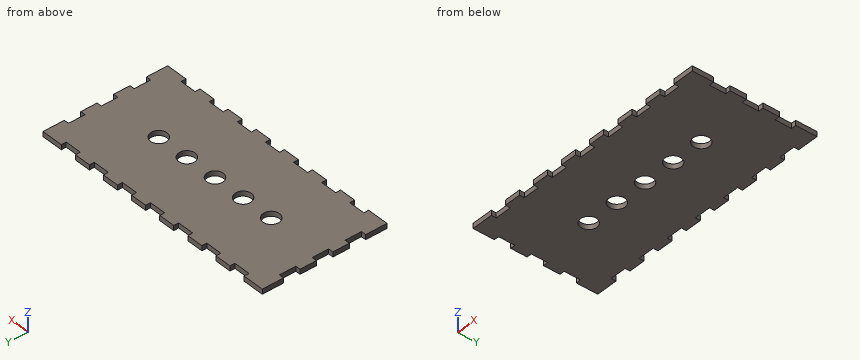
```python
from build123d import *

# Parameters (mm, degrees)
SKETCH1_R           = 5
BOSS_EXTRUDE1_DEPTH = 3


with BuildPart() as part:
    # Sketch1 → Boss-Extrude1 (new body)
    with BuildSketch(Plane.XY):
        Polygon((0, 60), (0, 50), (-3, 50), (-3, 40), (0, 40), (0, 30), (-3, 30), (-3, 20), (0, 20), (0, 10), (-3, 10), (-3, 0), (-3, -3), (0, -3), (10, -3), (10, 0), (20, 0), (20, -3), (30, -3), (30, 0), (40, 0), (40, -3), (50, -3), (50, 0), (60, 0), (60, -3), (70, -3), (70, 0), (80, 0), (80, -3), (90, -3), (90, 0), (100, 0), (100, -3), (110, -3), (110, 0), (120, 0), (120, -3), (130, -3), (130, 0), (140, 0), (140, -3), (150, -3), (153, -3), (153, 0), (153, 10), (150, 10), (150, 20), (153, 20), (153, 30), (150, 30), (150, 40), (153, 40), (153, 50), (150, 50), (150, 60), (153, 60), (153, 70), (153, 73), (150, 73), (140, 73), (140, 70), (130, 70), (130, 73), (120, 73), (120, 70), (110, 70), (110, 73), (100, 73), (100, 70), (90, 70), (90, 73), (80, 73), (80, 70), (70, 70), (70, 73), (60, 73), (60, 70), (50, 70), (50, 73), (40, 73), (40, 70), (30, 70), (30, 73), (20, 73), (20, 70), (10, 70), (10, 73), (0, 73), (-3, 73), (-3, 70), (-3, 60), align=None)
        with Locations((35, 35)):
            Circle(SKETCH1_R, mode=Mode.SUBTRACT)
        with Locations((55, 35)):
            Circle(SKETCH1_R, mode=Mode.SUBTRACT)
        with Locations((75, 35)):
            Circle(SKETCH1_R, mode=Mode.SUBTRACT)
        with Locations((95, 35)):
            Circle(SKETCH1_R, mode=Mode.SUBTRACT)
        with Locations((115, 35)):
            Circle(SKETCH1_R, mode=Mode.SUBTRACT)
    extrude(amount=BOSS_EXTRUDE1_DEPTH)


solid = part.part
```
Can you work these out from the model? Positions are in its coordinate system, mm. Give positions to 0.01 mm unless a question says otherwise; leave off trailing zeros. Loops run counter-clockwise (first coordinate to the right, second up) from the corner with the lowest first, then second, coordinate; pieces in that order, holes last. Notation, with made-up numbers: M 20,87.25 L 62,87.25 A19 cw 62,115.25 Z; hole C -28,-27 d1. An arc over 180 degrees is marked long. Use one line per item in the form item = value. Start each with the question number.
(1) I want a section at A-A, the plane x = 95. Write out the boundary of the cut face in (y, z), and give its area (3 significant figures).
(2) Please list where these lines run through material, in increasing order: line 1 (Y direction, x = 55, z = 1.2); line 2 (X direction, y = 32, z = 1.8); line 3 (X direction, y = 52.5, z = 2.6).
(3) I'm going to push flat-ended pins straight in: P1, Ø0.9, axis at x = 53, z = 1, coming from the +Y side; P2, Ø0.9, axis at x = 93.5, z = 1, coming from the -Y side. Where does each tip first touch, or does it pass through?
(4) I want a section at B-B, the plane y = 35. Write out the boundary of the cut face in (x, z), and give its area (3 significant figures).
(5) I want a section at C-C, the plane z = 1.25. State how many separate pieces and enclosed holes the cut face has, and give its area (3 significant figures).
(6) I want a section at D-D, the plane x = 38.5. Write out the boundary of the cut face in (y, z), and give its area (3 significant figures).
Worked out:
q1.outline = M 0,0 L 30,0 L 30,3 L 0,3 Z; M 40,0 L 70,0 L 70,3 L 40,3 Z
q1.area = 180 mm²
q2.line_1 = 0 to 30, 40 to 70
q2.line_2 = 0 to 31, 39 to 51, 59 to 71, 79 to 91, 99 to 111, 119 to 150
q2.line_3 = 0 to 150
q3.P1 = 70
q3.P2 = 0
q4.outline = M 0,0 L 30,0 L 30,3 L 0,3 Z; M 40,0 L 50,0 L 50,3 L 40,3 Z; M 60,0 L 70,0 L 70,3 L 60,3 Z; M 80,0 L 90,0 L 90,3 L 80,3 Z; M 100,0 L 110,0 L 110,3 L 100,3 Z; M 120,0 L 150,0 L 150,3 L 120,3 Z
q4.area = 300 mm²
q5.separate_pieces = 1
q5.enclosed_holes = 5
q5.area = 10,900 mm²
q6.outline = M 0,0 L 31.43,0 L 31.43,3 L 0,3 Z; M 38.57,0 L 70,0 L 70,3 L 38.57,3 Z
q6.area = 189 mm²
